The figure shows three views and two pictorial views of one solid part (mm, origin at its lowest corner). Answer the questions. A direction names the side the tool comes from. Coordinates: 2 decimals unless noted, no trailing zeros. Write each loop counter-clockwise with the first axis right and the second up, starting at its lowest first coordinate (ties: lowest second). Pieces come first, ordered by that corner, then holes. Notation, with made-up numbers: M 28.25,36.5 L 86.25,36.5 A16 cw 86.25,62.5 Z; hole C -26.5,-39.75 d3. An arc over 180 degrees is marked long. Use a Markdown table: item, result. Add a question column.
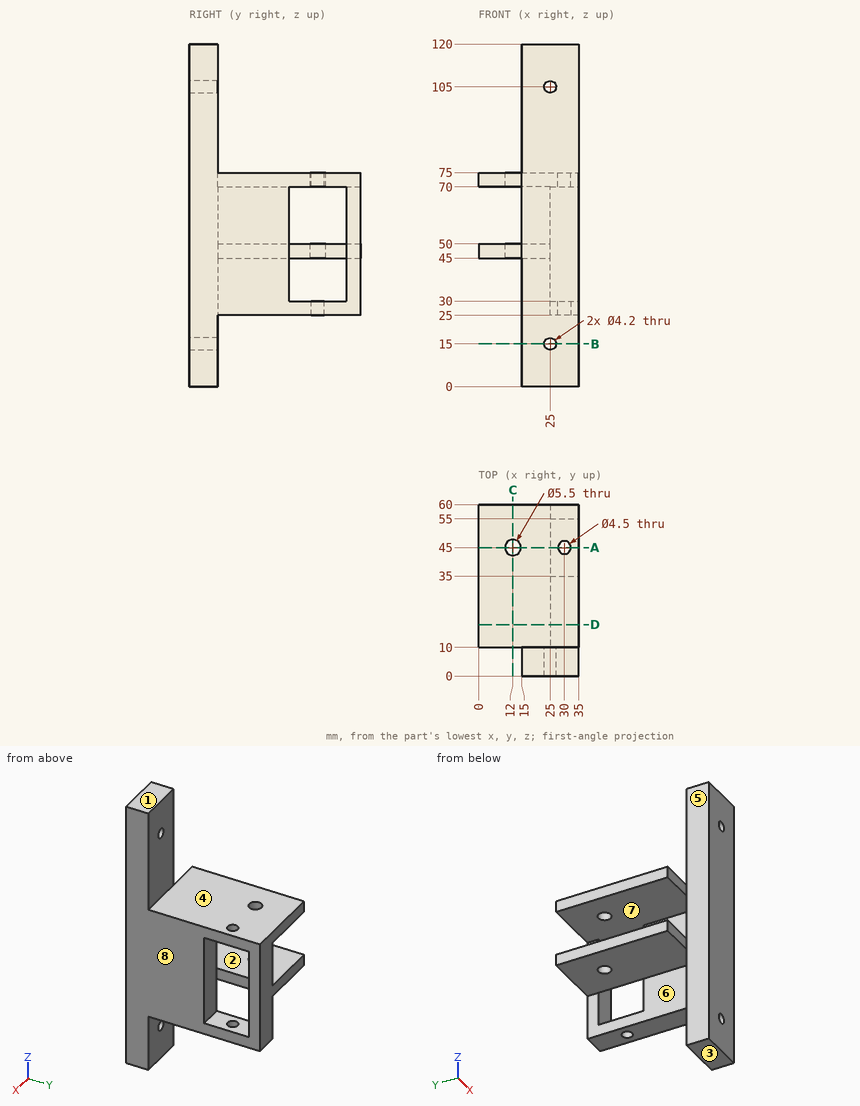
Item 1: Find section C-C on x = 12. Give the vertices of the cut face in (y, z), then the cut area to 3 significant figures.
Item 2: Find section A-A on y = 45. Give the vertices of the cut face in (x, z).
Item 3: Find section D-D on y = 18. Give the vertices of the cut face in (x, z), then the cut area to 3 significant figures.
Item 4: Each of these flat-tipped pins is pushed along its axis until it touches: pin 1 (10 mm diameter, centred on x = 28, z = 14.5, fed in from +Y); pin 2 (8 mm diameter, centred on y = 11, z = 26.5, fed in from -X); pin 3 (6.5 mm diameter, centred on x = 12, y = 45, fed in from -Z); pin 4 (2.5 mm diameter, centred on x = 30, y = 45, fed in from -Z). Where does it stop, or does it pass through?
Item 5: Find section B-B on z = 15. Give the vertices of the cut face in (x, y), then the cut area to 3 significant figures.
Item 6: Determine the mould class of the marked faces 1, 2 and 3 for opening direction Z: pulls with the +Z half, pulls with the -Z half, needs draft (parallel to the pull), parting line crosses it, or undercut.
Item 7: For the marked faces 4, 5, 6, 7 and 8, determine the directions among +Z, -Z, +X, -X, +Y, -Y from which every point of the face is accessible in a straight line to the end or side of a thin tool.
Item 8: Consider probe 1 along Z at (x, y) = (2.5, 43); probe 2 along Y at (x, z) = (12, 48); probe 3 along Y at (x, z) = (30, 28). Determine where each line is inside the solid, lowest interval first.
Geometry says:
| question | item | result |
|---|---|---|
| 1 | outline | M 10,45 L 42.25,45 L 42.25,50 L 10,50 Z; M 10,70 L 42.25,70 L 42.25,75 L 10,75 Z; M 47.75,45 L 60,45 L 60,50 L 47.75,50 Z; M 47.75,70 L 60,70 L 60,75 L 47.75,75 Z |
| 1 | area | 445 mm2 |
| 2 | outline | M 0,45 L 9.25,45 L 9.25,50 L 0,50 Z; M 0,70 L 9.25,70 L 9.25,75 L 0,75 Z; M 14.75,45 L 25,45 L 25,50 L 14.75,50 Z; M 14.75,70 L 27.75,70 L 27.75,75 L 14.75,75 Z; M 25,25 L 27.75,25 L 27.75,30 L 25,30 Z; M 32.25,25 L 35,25 L 35,30 L 32.25,30 Z; M 32.25,70 L 35,70 L 35,75 L 32.25,75 Z |
| 3 | outline | M 0,45 L 25,45 L 25,25 L 35,25 L 35,75 L 0,75 L 0,70 L 25,70 L 25,50 L 0,50 Z |
| 3 | area | 750 mm2 |
| 4 | pin 1 | stops at y = 10 |
| 4 | pin 2 | stops at x = 15 |
| 4 | pin 3 | stops at z = 45 |
| 4 | pin 4 | passes through |
| 5 | outline | M 15,0 L 22.9,0 L 22.9,10 L 15,10 Z; M 27.1,0 L 35,0 L 35,10 L 27.1,10 Z |
| 5 | area | 158 mm2 |
| 6 | face 1 | pulls with the +Z half |
| 6 | face 2 | undercut |
| 6 | face 3 | pulls with the -Z half |
| 7 | face 4 | +Z, +X, -X, +Y |
| 7 | face 5 | +Z, -Z, -X, -Y |
| 7 | face 6 | -Z, -X, +Y |
| 7 | face 7 | -X |
| 7 | face 8 | +Z, -Z, +X, +Y, -Y |
| 8 | probe 1 | z = 45 to 50, 70 to 75 |
| 8 | probe 2 | y = 10 to 42.25, 47.75 to 60 |
| 8 | probe 3 | y = 0 to 42.75, 47.25 to 60 |
